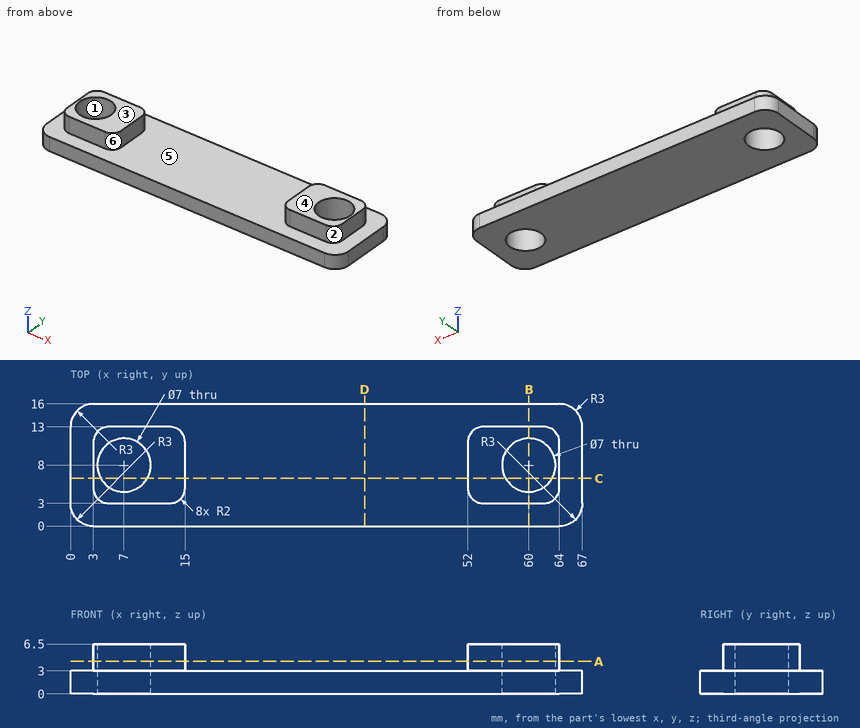
Drawing for the job (mm, zero at the part's lowest x, y, z). A direction names the side the tool comes from. Round coordinates to 2 decimals unless told otherwise and drop trailing zeros. Order: outer loops, then holes, each group sorted by start corner. A loop starts at its lowest first (then second) coordinate and runs counter-clockwise, first axis right, second up.
Item 1: Saw through at D-D on x = 38.5. Write the cut outline in (y, z).
Item 2: Saw through at C-C on y = 6.25. Write the cut outline in (x, z), then the cut area to 3 significant figures.
Item 3: Saw through at A-A on z = 4.25. Write the cut outline in (x, y).
Item 4: Mould opens along X. For the marked faces 1, 2 and 3 say: pulls with the +X half, pulls with the -X half, needs draft (parallel to the pull), parting line crosses it, or undercut.
Item 5: Probe line 1 along X through (y, z) = (5, 3.75); line 2 along Y through (x, z) = (7, 4.75); line 3 along Z through (x, y) = (38.5, 8). List the from-to ranges inside material, lowest first.
Item 6: Saw through at B-B on x = 60. Write the cut outline in (y, z).
Item 7: Pin check, flat tips, straight feed: pin 1 (3 mm diameter, centred on y = 8.5, z = 5, fed in from -X); pin 2 (3 mm diameter, centred on x = 9, z = 5, fed in from +Y); pin 3 (1 mm diameter, centred on x = 56.5, z = 5, fed in from -Y). Stop position of each tip, or through.
Item 8: Tool access for the marked faces 4, 5 and 6: list every direction of +Z, -Z, +X, -X, +Y, -Y with a clear straight run to the whole face (end or side of a thin tool).
Reported:
1. outline: (0, 0) - (16, 0) - (16, 3) - (0, 3) - close
2. outline: (0, 0) - (3.97, 0) - (3.97, 6.5) - (3, 6.5) - (3, 3) - (0, 3) - close; (10.03, 0) - (56.97, 0) - (56.97, 6.5) - (52, 6.5) - (52, 3) - (15, 3) - (15, 6.5) - (10.03, 6.5) - close; (63.03, 0) - (67, 0) - (67, 3) - (64, 3) - (64, 6.5) - (63.03, 6.5) - close
2. area: 206 mm2
3. outline: (3, 5) arc R2 ccw to (5, 3) - (13, 3) arc R2 ccw to (15, 5) - (15, 11) arc R2 ccw to (13, 13) - (5, 13) arc R2 ccw to (3, 11) - close; (52, 5) arc R2 ccw to (54, 3) - (62, 3) arc R2 ccw to (64, 5) - (64, 11) arc R2 ccw to (62, 13) - (54, 13) arc R2 ccw to (52, 11) - close; hole circle Ø7 at (7, 8); hole circle Ø7 at (60, 8)
4. face 1: undercut
4. face 2: pulls with the +X half
4. face 3: needs draft
5. line 1: x = 3 to 5.2, 8.8 to 15, 52 to 58.2, 61.8 to 64
5. line 2: y = 3 to 4.5, 11.5 to 13
5. line 3: z = 0 to 3
6. outline: (0, 0) - (4.5, 0) - (4.5, 6.5) - (3, 6.5) - (3, 3) - (0, 3) - close; (11.5, 0) - (16, 0) - (16, 3) - (13, 3) - (13, 6.5) - (11.5, 6.5) - close
7. pin 1: stops at x = 3
7. pin 2: stops at y = 13
7. pin 3: stops at y = 3
8. face 4: +Z, +X, -X, +Y, -Y
8. face 5: +Z
8. face 6: +Z, -Y
